```python
from build123d import *

# Parameters (mm, degrees)
SKETCH_1_W          = 8
SKETCH_1_H          = 11.8
EXTRUDE_1_DEPTH     = 3.8
FILLET_1_R          = 4
CUT_EXTRUDE_1_DEPTH = 0.35


with BuildPart() as part:
    # 草圖1 → 填料-伸長1 (new body)
    with BuildSketch(Plane(origin=(0, 0, 0), x_dir=(1, 0, 0), z_dir=(0, 1, 0))):
        with Locations((4, 5.9)):
            Rectangle(SKETCH_1_W, SKETCH_1_H)
    extrude(amount=EXTRUDE_1_DEPTH)

    # 圓角1
    fillet_1_edges = [part.edges().sort_by_distance(p)[0] for p in [
        (8, 1.9, -11.8),
        (8, 1.9, 0),
    ]]
    fillet(fillet_1_edges, radius=FILLET_1_R)

    # 草圖2 → 除料-伸長1 (cut, symmetric)
    with BuildSketch(Plane(origin=(0, 1.8, 0), x_dir=(1, 0, 0), z_dir=(0, 1, 0))):
        with BuildLine():
            Line((0, 11.8), (0, 11.025723127))
            Line((0, 11.025723127), (4.903996853, 11.025723127))
            ThreePointArc((4.903996853, 11.025723127), (6.669352867, 9.824118394), (7.35, 7.8))
            Line((7.35, 7.8), (7.35, 4))
            ThreePointArc((7.35, 4), (6.637408845, 1.934431172), (4.802791293, 0.74761224))
            Line((4.802791293, 0.74761224), (0, 0.65))
            Line((0, 0.65), (0, 0))
            Line((0, 0), (4, 0))
            ThreePointArc((4, 0), (6.828427125, 1.171572875), (8, 4))
            Line((8, 4), (8, 7.8))
            ThreePointArc((8, 7.8), (6.828427125, 10.628427125), (4, 11.8))
            Line((4, 11.8), (0, 11.8))
        make_face()
    extrude(amount=CUT_EXTRUDE_1_DEPTH, both=True, mode=Mode.SUBTRACT)


solid = part.part
```
CAD build for the part. Positions are in the model's coordinates, mm. A direction names the side the tool comes from. Give positions to 0.01 mm unless a question says otherwise; leave off trailing zeros. Loops run counter-clockwise (first coordinate to the right, second up) from the corner with the lowest first, then second, coordinate; pieces in that order, holes last. Notation, with made-up numbers: M -39,27 L 7,27 A10 cw 7,34 Z; hole C 11,50 d7. An arc over 180 degrees is marked long. Use one line per item in the form item = value.
Item 1: Drill centre lines: probe 1 along X at (y, z) = (1.5, -6.5); probe 2 along Z at (x, y) = (5.5, 1.8); probe 3 along Z at (x, y) = (6.5, 0.8). Where is each one in solid material? Low to high. Write a range as from..to.
Determined:
probe_1 = 0..7.35
probe_2 = -10.8..-1
probe_3 = -10.92..-0.88
Item 2: Slice it at A-A (y = 3.4). List the corners of the cut face in (x, z), plus the area to 3 significant figures.
Determined:
outline = M 0,-11.8 L 4,-11.8 A4 ccw 8,-7.8 L 8,-4 A4 ccw 4,0 L 0,0 Z
area = 87.5 mm2
Item 3: Flat gauge pins, fed straight in: pin 1 (1 mm diameter, centred on x = 6.5, y = 3, fed in from +Z); pin 2 (4 mm diameter, centred on x = 2.5, z = -3, fed in from -Y); pin 3 (1 mm diameter, centred on x = 6, y = 3, fed in from -Z); pin 4 (2 mm diameter, centred on x = 5.5, y = 2, fed in from -Z). Where does each tip first touch, or does it go through?
Determined:
pin_1 = -0.54
pin_2 = 0
pin_3 = -11.51
pin_4 = -11.77
Item 4: Slice it at D-D (y = 1.85). List the corners of the cut face in (x, z), plus the area to 3 significant figures.
Determined:
outline = M 0,-11.03 L 4.9,-11.03 A3.35 ccw 7.35,-7.8 L 7.35,-4 A3.35 ccw 4.8,-0.75 L 0,-0.65 Z
area = 71.6 mm2
Item 5: Two-plate mould, pull along Y, no slides. Class faces 4 (the face through (6.65, 1.8, -9.85)), 5 (the face through (8, 1, -6)), 6 (the face through (4, 3.8, -6)): pulls with the +Y half, pulls with the -Y half, needs draft (parallel to the pull), parting line crosses it, or undercut.
Determined:
face_4 = undercut
face_5 = needs draft
face_6 = pulls with the +Y half
Item 6: Slice it at C-C (x = 1.5). List the corners of the cut face in (y, z), plus the area to 3 significant figures.
Determined:
outline = M 0,-11.8 L 1.45,-11.8 L 1.45,-11.03 L 2.15,-11.03 L 2.15,-11.8 L 3.8,-11.8 L 3.8,0 L 2.15,0 L 2.15,-0.68 L 1.45,-0.68 L 1.45,0 L 0,0 Z
area = 43.8 mm2
Item 7: Slice it at B-B (z = -8.5). List the corners of the cut face in (x, y), plus the area to 3 significant figures.
Determined:
outline = M 0,0 L 7.94,0 L 7.94,1.45 L 7.28,1.45 L 7.28,2.15 L 7.94,2.15 L 7.94,3.8 L 0,3.8 Z
area = 29.7 mm2
Item 8: Which spindle directions (+Z, -Z, +X, -X, +Y, -Y) get a long thin tool onto all of the face, cutting with end or side? Do faces 1 (the face through (7.5, 1.45, -5.9)), 2 (the face through (6.859, 2.987, -10.597)), 3 (the face through (6.657, 1.805, -1.959)). Say none if no direction does.
Determined:
face_1 = +X
face_2 = -Z, +X, +Y, -Y
face_3 = +Z, +X
